```python
from build123d import *

# Parameters (mm, degrees)
SKETCH1_W                                        = 100
SKETCH1_H                                        = 110
BOSS_EXTRUDE2_DEPTH                              = 12.7
CSK_FOR_1_4_FLAT_HEAD_MACHINE_SCREW3_D           = 6.5278
CSK_FOR_1_4_FLAT_HEAD_MACHINE_SCREW3_CSINK_D     = 12.8778
CSK_FOR_1_4_FLAT_HEAD_MACHINE_SCREW3_CSINK_ANGLE = 82
CSK_FOR_1_4_FLAT_HEAD_MACHINE_SCREW4_D           = 6.5278
CSK_FOR_1_4_FLAT_HEAD_MACHINE_SCREW4_CSINK_D     = 12.8778
CSK_FOR_1_4_FLAT_HEAD_MACHINE_SCREW4_CSINK_ANGLE = 82
FILLET1_R                                        = 2
CUT_EXTRUDE1_DEPTH                               = 150.202178268


with BuildPart() as part:
    # Sketch1 → Boss-Extrude2 (new body)
    with BuildSketch(Plane.XY):
        with Locations((50, -55)):
            Rectangle(SKETCH1_W, SKETCH1_H)
        Polygon((70, -39.025625978), (76.45, -39.025625978), (76.25, -55), (76.25, -70.975625978), (70, -70.975625978), (63.55, -70.975625978), (63.55, -39.025625978), align=None, mode=Mode.SUBTRACT)
    extrude(amount=BOSS_EXTRUDE2_DEPTH)

    # CSK for 1/4 Flat Head Machine Screw3 (through all)
    with Locations(Plane(origin=(0, 0, 0), x_dir=(-1, 0, 0), z_dir=(0, 0, -1))):
        with Locations((-70, -90.31)):
            CounterSinkHole(CSK_FOR_1_4_FLAT_HEAD_MACHINE_SCREW3_D / 2, CSK_FOR_1_4_FLAT_HEAD_MACHINE_SCREW3_CSINK_D / 2, counter_sink_angle=CSK_FOR_1_4_FLAT_HEAD_MACHINE_SCREW3_CSINK_ANGLE)

    # CSK for 1/4 Flat Head Machine Screw4 (through all)
    with Locations(Plane(origin=(0, 0, 0), x_dir=(-1, 0, 0), z_dir=(0, 0, -1))):
        with Locations((-70, -19.69)):
            CounterSinkHole(CSK_FOR_1_4_FLAT_HEAD_MACHINE_SCREW4_D / 2, CSK_FOR_1_4_FLAT_HEAD_MACHINE_SCREW4_CSINK_D / 2, counter_sink_angle=CSK_FOR_1_4_FLAT_HEAD_MACHINE_SCREW4_CSINK_ANGLE)

    # Fillet1
    fillet1_edges = [part.edges().sort_by_distance(p)[0] for p in [
        (0, 0, 6.35),
        (100, 0, 6.35),
        (100, -110, 6.35),
        (0, -110, 6.35),
    ]]
    fillet(fillet1_edges, radius=FILLET1_R)

    # Sketch15 → Cut-Extrude1 (cut, through all)
    with BuildSketch(Plane(origin=(0, 0, 0), x_dir=(-1, 0, 0), z_dir=(0, 0, -1))):
        with BuildLine():
            Line((-56.200253658, -14.19), (-6.200253658, -14.19))
            ThreePointArc((-6.200253658, -14.19), (-2.900253658, -17.49), (-6.200253658, -20.79))
            Line((-6.200253658, -20.79), (-56.200253658, -20.79))
            ThreePointArc((-56.200253658, -20.79), (-59.500253658, -17.49), (-56.200253658, -14.19))
        make_face()
        with BuildLine():
            Line((-56.200253658, -89.21), (-6.200253658, -89.21))
            ThreePointArc((-6.200253658, -89.21), (-2.900253658, -92.51), (-6.200253658, -95.81))
            Line((-6.200253658, -95.81), (-56.200253658, -95.81))
            ThreePointArc((-56.200253658, -95.81), (-59.500253658, -92.51), (-56.200253658, -89.21))
        make_face()
    extrude(amount=-CUT_EXTRUDE1_DEPTH, mode=Mode.SUBTRACT)


solid = part.part
```
Design review of the part built by this model. Coordinates are the model's own, in mm. A direction names the side the tool comes from. Coordinates: 2 decimals unless noted, no trailing zeros. Loops run counter-clockwise (first coordinate to the right, second up) from the corner with the lowest first, then second, coordinate; pieces in that order, holes last.
Q1. We need section D-D on z = 5.25. State the section outline as (x, y) points.
Reported:
outline: (0, -108) arc R2 ccw to (2, -110) - (98, -110) arc R2 ccw to (100, -108) - (100, -2) arc R2 ccw to (98, 0) - (2, 0) arc R2 ccw to (0, -2) - close; hole (6.2, -95.81) - (56.2, -95.81) arc R3.3 ccw to (56.2, -89.21) - (6.2, -89.21) arc R3.3 ccw to start; hole (6.2, -20.79) - (56.2, -20.79) arc R3.3 ccw to (56.2, -14.19) - (6.2, -14.19) arc R3.3 ccw to start; hole (63.55, -70.98) - (76.25, -70.98) - (76.25, -55) - (76.45, -39.03) - (63.55, -39.03) - close; hole circle Ø6.53 at (70, -90.31); hole circle Ø6.53 at (70, -19.69)
Q2. Tool access review of faces 4 (the face through (49, -54, 12.7)), 5 (the face through (2.9, -17.4, 6.3)): name each direction out of +Z, -Z, +X, -X, +Y, -Y from which nothing blocks a thin tool from reaching the whole face with its end or side.
Reported:
face 4: +Z, +X, -X, +Y, -Y
face 5: +Z, -Z
Q3. We need section A-A on x = 70. State the section outline as (y, z) points, and give its area (3 significant figures).
Reported:
outline: (-110, 0) - (-96.75, 0) - (-93.57, 3.65) - (-93.57, 12.7) - (-110, 12.7) - close; (-87.05, 3.65) - (-83.87, 0) - (-70.98, 0) - (-70.98, 12.7) - (-87.05, 12.7) - close; (-39.03, 0) - (-26.13, 0) - (-22.95, 3.65) - (-22.95, 12.7) - (-39.03, 12.7) - close; (-16.43, 3.65) - (-13.25, 0) - (0, 0) - (0, 12.7) - (-16.43, 12.7) - close
area: 802 mm2
Q4. The part is to be moulded in two halves that separate along Y. For faces 1 (the face through (49, 0, 6)), 2 (the face through (69.3, -93.5, 8.2)), 3 (the face through (49, -54, 0)), say which applies: +Y half, -Y half, draft (parallel to the pull), parting line (faces both ways), or undercut.
Reported:
face 1: +Y half
face 2: undercut
face 3: draft
Q5. We need section B-B on x = 34. State the section outline as (y, z) points, and give its area (3 significant figures).
Reported:
outline: (-110, 0) - (-95.81, 0) - (-95.81, 12.7) - (-110, 12.7) - close; (-89.21, 0) - (-20.79, 0) - (-20.79, 12.7) - (-89.21, 12.7) - close; (-14.19, 0) - (0, 0) - (0, 12.7) - (-14.19, 12.7) - close
area: 1,230 mm2
Q6. We need section C-C on y = -68.5. State the section outline as (x, z) points.
Reported:
outline: (0, 0) - (63.55, 0) - (63.55, 12.7) - (0, 12.7) - close; (76.25, 0) - (100, 0) - (100, 12.7) - (76.25, 12.7) - close
Q7. To check wall thickness, follow line 1 (Y direction, x = 70, z = 9.75); line 2 (Y direction, x = 40, z = 6); line 3 (X direction, y = -60, z = 11.5). State the ranges of each line that lie inside material, in increasing order.
Reported:
line 1: y = -110 to -93.57, -87.05 to -70.98, -39.03 to -22.95, -16.43 to 0
line 2: y = -110 to -95.81, -89.21 to -20.79, -14.19 to 0
line 3: x = 0 to 63.55, 76.25 to 100
